Work out the finished part from the listing and answer in its coordinate system (mm). A direction names the side the tool comes from. Round coordinates to 2 decimals unless told otherwise and drop trailing zeros. Loops run counter-clockwise (first coordinate to the right, second up) from the corner with the lowest first, then second, coordinate; pieces in that order, holes last. Notation, with made-up numbers: (85.25, 65) -> (121.25, 65) arc R11 ccw to (121.25, 84) -> close; hole circle Ø4 at (0, 29.5). An arc over 180 degrees is marked (long way). Use one line per item in the form item = value.
```python
from build123d import *

# Parameters (mm, degrees)
SKETCH5_R     = 9.55
STUB_DEPTH    = 37.5
BORE_SKETCH_R = 7.85
BORE_DEPTH    = 46.276925691


with BuildPart() as part:
    # Sketch1 → Flange (revolve)
    with BuildSketch(Plane(origin=(0, 0, 0), x_dir=(0, 0, -1), z_dir=(1, 0, 0)), mode=Mode.PRIVATE) as flange_sk:
        Polygon((-15, 0), (-15, 3.2), (-6.789488223, 5.4), (0, 5.4), (0, 2.5), (-8.1, 2.5), (-8.1, 0), align=None)
    revolve(flange_sk.sketch.rotate(Axis((0, 0, 0), (0, 1, 0)), 180), axis=Axis((0, 0, 0), (0, 1, 0)))

    # Sketch5 → Stub (add)
    with BuildSketch(Plane.XZ.offset(-2.5)):
        with Locations(Location((0, 0, 0), (0, 0, 270))):
            Circle(SKETCH5_R)
    extrude(amount=-STUB_DEPTH)

    # Bore Sketch → Bore (cut, through all)
    with BuildSketch(Plane(origin=(0, 40, 0), x_dir=(1, 0, 0), z_dir=(0, 1, 0))):
        with Locations(Location((0, 0, 0), (0, 0, 270))):
            Circle(BORE_SKETCH_R)
    extrude(amount=-BORE_DEPTH, mode=Mode.SUBTRACT)


solid = part.part
```
(1) For faces 4 (the cylindrical face through (7.907, 1.232, 1.756)), 5 (the flat face through (-8, 40, 1)), 6 (the cylindrical face through (2.9, 22.1, -9.1)), determine the directions among +Z, -Z, +X, -X, +Y, -Y from which every point of the face is accessible in a straight line to the end or side of a thin tool.
Completed:
face_4 = -Y
face_5 = +Z, -Z, +X, -X, +Y
face_6 = +Y
(2) For a pull along X with two mould halves and no side action, classify faces 1 (the flat face through (6, 0, 6)), 2 (the cylindrical face through (-12.65, 1.62, -8.06)), 3 (the cylindrical face through (-4.777, 21.512, -6.229)) as +X half, -X half, draft (parallel to the pull), parting line (faces both ways), or undercut.
Completed:
face_1 = draft
face_2 = parting line
face_3 = undercut
(3) Find section A-A, the plane x = 0. Write down the section's boundary in (y, z).
Completed:
outline = (0, -15) -> (3.2, -15) -> (4.66, -9.55) -> (40, -9.55) -> (40, -7.85) -> (2.5, -7.85) -> (2.5, -8.1) -> (0, -8.1) -> close; (0, 8.1) -> (2.5, 8.1) -> (2.5, 7.85) -> (40, 7.85) -> (40, 9.55) -> (4.66, 9.55) -> (3.2, 15) -> (0, 15) -> close
(4) Find section B-B, the plane z = 0. Write down the section's boundary in (x, y), then the cut area to 3 significant figures.
Completed:
outline = (-15, 0) -> (-8.1, 0) -> (-8.1, 2.5) -> (-7.85, 2.5) -> (-7.85, 40) -> (-9.55, 40) -> (-9.55, 4.66) -> (-15, 3.2) -> close; (7.85, 2.5) -> (8.1, 2.5) -> (8.1, 0) -> (15, 0) -> (15, 3.2) -> (9.55, 4.66) -> (9.55, 40) -> (7.85, 40) -> close
area = 178 mm2
(5) Find section C-C, the plane y = 37.5. Write down the section's boundary in (x, z).
Completed:
outline = circle Ø19.1 at (0, 0); hole circle Ø15.7 at (0, 0)
(6) Consider L1, parallel to X at y = 7, z = 0; L2, parallel to X at y = 1.9, z = 0; L3, parallel to Z at x = -4.5, y = 17.5. Determine where each line is inside the solid, lowest interval first.
Completed:
L1 = -9.55 to -7.85, 7.85 to 9.55
L2 = -15 to -8.1, 8.1 to 15
L3 = -8.42 to -6.43, 6.43 to 8.42
(7) Given P1, Ø9.5, axis at x = 0, z = 0, coming from the +Y side; P2, Ø8, axis at y = 4, z = -8.5, coming from the -X side; P3, Ø6, axis at y = 15, z = 7, coming from the +X side; P4, Ø5, axis at x = -10.5, y = 22.5, coming from the +Z side, each flat-ended and moving along its own axis, determine where each tip first touches the part or whether it passes through.
Completed:
P1 = through
P2 = -14.28
P3 = 8.67
P4 = 5.22
